Autodesk Inventor part; units mm, degrees
ref_plane "YZ Plane" through (0, 0, 0) normal (1, 0, 0) x (0, 1, 0)
ref_plane "XZ Plane" through (0, 0, 0) normal (0, 1, 0) x (-1, 0, 0)
ref_plane "XY Plane" through (0, 0, 0) normal (0, 0, 1) x (1, 0, 0)
sketch "Sketch_1" plane through (0, 0, 0) normal (0, 0, 1) x (1, 0, 0)
  line L0 (582, 0) -> (0, 0)
  line L1 (0, 0) -> (0, 4.5)
  line L2 (0, 4.5) -> (0.5, 5)
  line L3 (0.5, 5) -> (581.5, 5)
  line L4 (581.5, 5) -> (582, 4.5)
  line L5 (582, 4.5) -> (582, 0)
  line L6 (582, 0) -> (0, 0)
revolve "Revolution1" add sketch "Sketch_1" angle 360 about axis through (582, 0, 0) along (1, 0, 0)
sketch "Sketch2" plane through (0, 0, 0) normal (-1, 0, 0) x (0, 0, 1)
  point P0 (0, 0)
hole "Hole1" at (0, 0, 0) direction (1, 0, 0) diameter 4.917 depth 17.5806 tip angle 120 countersink diameter 6 countersink angle 90
sketch "Sketch3" plane through (582, 0, 0) normal (1, 0, 0) x (0, 0, -1)
  point P0 (0, 0)
hole "Hole2" at (582, 0, 0) direction (-1, 0, 0) diameter 4.917 depth 17.5806 tip angle 120 countersink diameter 6 countersink angle 90
properties part number "PSSFGW10-582-M6-N6"
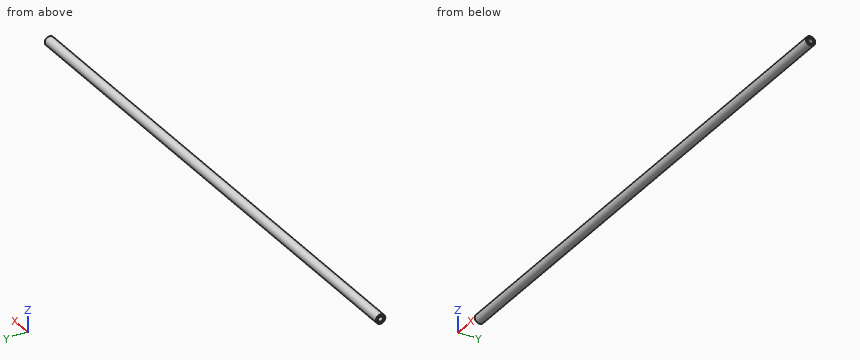
Part model, mm, in its own coordinate system. Give positions to 0.01 mm unless a question says otherwise; leave off trailing zeros. Order: outer loops, then holes, each group sorted by start corner. A loop starts at its lowest first (then second) coordinate and runs counter-clockwise, first axis right, second up. Notation, with made-up numbers: (12.5, 87.25) - (25.5, 87.25) arc R32 cw to (25.5, 123.25) - close; hole circle Ø9 at (33, 17). An arc over 180 degrees is marked (long way). One line per question, with ' | ' between items.
1. Drill centre lines: probe 1 along Z at (x, y) = (10, 0); probe 2 along X at (y, z) = (2.25, 0.75); probe 3 along Y at (x, z) = (330, -2). Where is each one in solid material? Low to high.
Filled in:
probe 1: -5 to -2.46, 2.46 to 5 | probe 2: 17.63 to 564.37 | probe 3: -4.58 to 4.58
2. Band-saw the part on A-A on x = 426.5. List the corners of the cut face in (y, z).
Filled in:
outline: circle Ø10 at (0, 0)
3. Drop flat-ended pins along their axis: P1, Ø3, axis at x = 279, y = -3, coming from the -Z side; P2, Ø4.5, axis at y = 0, z = 0, coming from the -X side; P3, Ø4, axis at x = 77, z = 3, coming from the -Y side. Give the stop position or say it passes through.
Filled in:
P1: z = -4.77 | P2: x = 17.7 | P3: y = -4.9
